from build123d import *

# Parameters (mm, degrees)
SKETCH1_W                = 30.48
SKETCH1_H                = 16.51
BOSS_EXTRUDE1_DEPTH      = 2.54
BOSS_EXTRUDE2_DEPTH      = 10.16
BOSS_EXTRUDE2_DEPTH_BACK = 2.54
SKETCH3_W                = 30.48
SKETCH3_H                = 1.27
SKETCH4_W                = 30.48
SKETCH4_H                = 30.48
BOSS_EXTRUDE3_DEPTH      = 2.54
BODY_MOVE_COPY3_ANGLE    = 70
LOFT2_START              = -14.571578947
LOFT2_DEPTH              = 30.48
SKETCH5_R                = 2.159
CUT_EXTRUDE1_DEPTH       = 31.007586006
SKETCH6_W                = 30.48
SKETCH6_H                = 30.48
BOSS_EXTRUDE4_DEPTH      = 3.81


# Read off the part's stored shape, not the designer's step: Loft2
with BuildPart() as part:
    # Sketch1 → Boss-Extrude1 (new body)
    with BuildSketch(Plane(origin=(0, 0, 0), x_dir=(1, 0, 0), z_dir=(0, 1, 0))):
        with Locations((0.668421053, -1.938421053)):
            Rectangle(SKETCH1_W, SKETCH1_H)
    extrude(amount=BOSS_EXTRUDE1_DEPTH)

    # Sketch3 → Boss-Extrude2 (add, two sides: drawn at the far end of the back side and taken through both)
    with BuildSketch(Plane(origin=(0, 2.54, 0), x_dir=(1, 0, 0), z_dir=(0, 1, 0)).offset(-BOSS_EXTRUDE2_DEPTH_BACK)):
        with Locations((0.668421053, -10.828421053)):
            Rectangle(SKETCH3_W, SKETCH3_H)
    extrude(amount=BOSS_EXTRUDE2_DEPTH + BOSS_EXTRUDE2_DEPTH_BACK)


with BuildPart() as part_1:
    # Body-Move/Copy1: moved
    add(part.part.moved(Location((0, 7.62, 0))))


with BuildPart() as body_2:
    # Sketch4 → Boss-Extrude3 (new body)
    with BuildSketch(Plane(origin=(0, 0, 0), x_dir=(1, 0, 0), z_dir=(0, 1, 0))):
        with Locations((0.668421053, -3.843421053)):
            Rectangle(SKETCH4_W, SKETCH4_H)
    extrude(amount=BOSS_EXTRUDE3_DEPTH)


with BuildPart() as part_2:
    # Body-Move/Copy3: moved
    add(part_1.part.rotate(Axis((0, 13.97, 2.573421053), (1, 0, 0)), BODY_MOVE_COPY3_ANGLE))


    add(body_2.part)  # loft1 joins it to this body
    # loft from a face of the part (loft1)
    loft([part_2.faces().sort_by_distance((0.668421053, 5.616132601, 5.613980127))[0], part_2.faces().sort_by_distance((0.668421053, 2.54, 3.843421053))[0]])

    # Loft2 outline → Loft2 (add)
    with BuildSketch(Plane.YZ.offset(LOFT2_START)):
        Polygon((3.444304691, -0.353068015), (2.54, -11.396578947), (20.152039489, -6.434186164), align=None)
    extrude(amount=LOFT2_DEPTH)

    # Sketch5 → Cut-Extrude1 (cut, through all)
    with BuildSketch(Plane(origin=(0, 1.158164402, 3.182030543), x_dir=(1, 0, 0), z_dir=(0, 0.3420201433256677, 0.9396926207859089))):
        with Locations(Location((-8.856578947, 13.771344075, 0), (0, 0, 270))):
            Circle(SKETCH5_R)
        with Locations(Location((10.193421053, 13.771344075, 0), (0, 0, 270))):
            Circle(SKETCH5_R)
    extrude(amount=-CUT_EXTRUDE1_DEPTH, mode=Mode.SUBTRACT)

    # Sketch6 → Boss-Extrude4 (add)
    with BuildSketch(Plane.XZ):
        with Locations((0.668421053, 3.843421053)):
            Rectangle(SKETCH6_W, SKETCH6_H)
    extrude(amount=BOSS_EXTRUDE4_DEPTH)


solid = part_2.part
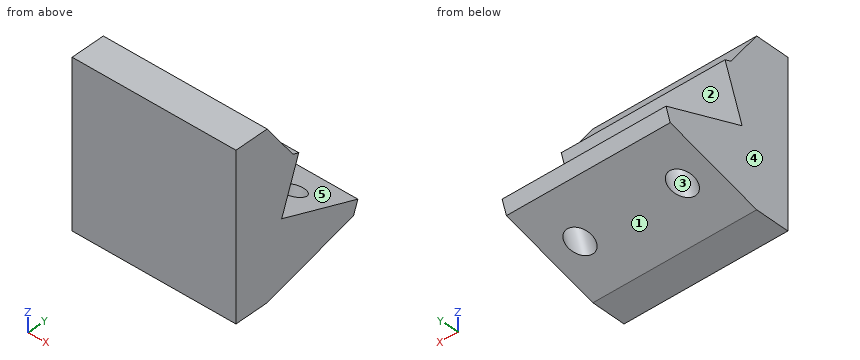
CAD build for the part. Positions are in the model's coordinates, mm. Face numbers are marked on the shaded views. A direction names the side the tool comes from. Give positions to 0.01 mm unless a question says otherwise; leave off trailing zeros. Loops run counter-clockwise (first coordinate to the right, second up) from the corner with the lowest first, then second, coordinate; pieces in that order, holes last. Notation, with made-up numbers: M 65.25,-15.5 L 98.25,-15.5 A11 cw 98.25,1.5 Z; hole C -17.75,18 d4. An arc over 180 degrees is marked long. Answer in a Markdown table with one row per item. Add a question column.
Item 1: Band-saw the part on C-C on z = 4.5. Give the cut face in (x, y).
Item 2: Band-saw the part on A-A on x = 8.5. Give the cut face in (y, z).
Item 3: Probe probe 1 along X at (y, z) = (13.5, -5.5); probe 2 along X at (y, z) = (12.5, -4.5); probe 3 along Z at (x, y) = (7, 14.5). List the from-to ranges inside material, lowest first.
Item 4: Mould opens along Y. For the marked faces 3, 4 and 5 say: +Y half, -Y half, draft (parallel to the pull), parting line (faces both ways), or undercut.
Item 5: Band-saw the part on D-D on y = 16.75. Give the cut face in (x, z), then the cut area to 3 significant figures.
Item 6: Band-saw the part on B-B on x = 5. Give the cut face in (y, z).
Item 7: Tool access for the marked faces 1 and 2: list every direction of +Z, -Z, +X, -X, +Y, -Y with a clear straight run to the whole face (end or side of a thin tool).
Reply:
| question | item | result |
|---|---|---|
| 1 | outline | M -14.57,-3.81 L 15.91,-3.81 L 15.91,6.56 L -14.57,6.56 Z |
| 2 | outline | M -3.81,-11.4 L 2.54,-11.4 L 9.83,-9.34 L 12.84,-1.07 L 5.51,1.6 L 8.98,11.15 L 7.79,11.58 L 2.54,19.08 L -3.81,19.08 Z; M 13.01,-8.45 L 20.15,-6.43 L 21.02,-4.05 L 15.36,-1.99 Z |
| 3 | probe 1 | x = -14.57 to -10.86, -6.85 to 8.19, 12.2 to 15.91 |
| 3 | probe 2 | x = -14.57 to -10.96, -6.75 to 8.09, 12.3 to 15.91 |
| 3 | probe 3 | z = -8.03 to -1.67 |
| 4 | face 3 | undercut |
| 4 | face 4 | draft |
| 4 | face 5 | +Y half |
| 5 | outline | M -14.57,-7.39 L 15.91,-7.39 L 15.91,-2.49 L -14.57,-2.49 Z |
| 5 | area | 149 mm^2 |
| 6 | outline | M -3.81,-11.4 L 2.54,-11.4 L 20.15,-6.43 L 21.02,-4.05 L 5.51,1.6 L 8.98,11.15 L 7.79,11.58 L 2.54,19.08 L -3.81,19.08 Z |
| 7 | face 1 | -Z, +X, -X, +Y |
| 7 | face 2 | +X, -X, +Y |
